Input: part model. Units: mm. Frame: model coordinates. Face numbers are marked on the shaded views. Give positions to 0.01 mm unless a question says otherwise; leave off trailing zeros. Loops run counter-clockwise (first coordinate to the right, second up) from the corner with the lowest first, then second, coordinate; pieces in that order, holes last. Notation, with made-up numbers: (32.5, 57.25) -> (71.5, 57.25) arc R29 cw to (71.5, 90.25) -> close; hole circle Ø5 at (-16, -27.75). An arc over 180 degrees is marked (long way). Answer in a Markdown table with one row per item. Add a question column.
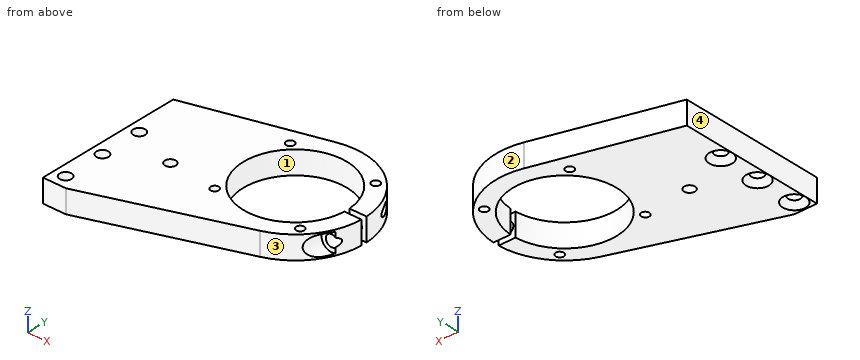
```python
from build123d import *

# Parameters (mm, degrees)
BOSS_EXTRUDE1_DEPTH         = 12.7
CUT_EXTRUDE1_DEPTH          = 13.7
SKETCH3_W                   = 28.575
SKETCH3_H                   = 12.7
F_8_CLEARANCE_HOLE1_D       = 4.5
F_8_CLEARANCE_HOLE1_DEPTH   = 12.7
F_1_4_CLEARANCE_HOLE1_D     = 6.6
F_1_4_CLEARANCE_HOLE1_DEPTH = 12.7
F_12_CLEARANCE_HOLE1_D      = 6
F_12_CLEARANCE_HOLE1_DEPTH  = 12.7
HOLE1_D                     = 6.4
HOLE1_DEPTH                 = 24.77643101
HOLE1_CBORE_D               = 11.2
HOLE1_CBORE_DEPTH           = 11.77643101
F_10_CLEARANCE_HOLE1_D      = 5
F_10_CLEARANCE_HOLE1_DEPTH  = 36.4125
CHAMFER1_SIZE               = 3
SKETCH14_R                  = 4
SKETCH14_R_2                = 3
BOSS_EXTRUDE2_DEPTH         = 12.7


with BuildPart() as part:
    # Sketch1 → Boss-Extrude1 (new body)
    with BuildSketch(Plane(origin=(0, 0, 0), x_dir=(-1, 0, 0), z_dir=(0, 0, -1))):
        with BuildLine():
            Line((224.169455465, 127.72254562), (151.435240745, 147.211619716))
            ThreePointArc((151.435240745, 147.211619716), (105.257753851, 121.607458019), (129.246532787, 74.570537656))
            Line((129.246532787, 74.570537656), (211.469455465, 46.304993078))
            Line((211.469455465, 46.304993078), (224.169455465, 46.304993078))
            Line((224.169455465, 46.304993078), (224.169455465, 127.72254562))
        make_face()
    extrude(amount=-BOSS_EXTRUDE1_DEPTH)

    # Sketch2 → Cut-Extrude1 (cut, through all)
    with BuildSketch(Plane.XY.offset(12.7)):
        with BuildLine():
            Line((-103.633291463, 112.093938317), (-113.179018515, 112.093938317))
            ThreePointArc((-113.179018515, 112.093938317), (-113.134717032, 110.506438317), (-113.179018515, 108.918938317))
            Line((-113.179018515, 108.918938317), (-103.633291463, 108.918938317))
            ThreePointArc((-103.633291463, 108.918938317), (-103.600117032, 110.506438317), (-103.633291463, 112.093938317))
        make_face()
    extrude(amount=-CUT_EXTRUDE1_DEPTH, mode=Mode.SUBTRACT)

    # Sketch3 → Cut-Revolve1 (revolve, cut)
    with BuildSketch(Plane(origin=(0, 110.506438317, 0), x_dir=(1, 0, 0), z_dir=(0, 1, 0))):
        with Locations((-127.312617032, -6.35)):
            Rectangle(SKETCH3_W, SKETCH3_H)
    revolve(axis=Axis((-141.600117032, 110.506438317, 0), (0, 0, 1)), mode=Mode.SUBTRACT)

    # #8 Clearance Hole1
    with Locations(Plane.XY.offset(12.7)):
        with Locations((-117.978117032, 86.884438317), (-165.222117032, 86.884438317), (-165.222117032, 134.128438317), (-117.978117032, 134.128438317)):
            Hole(F_8_CLEARANCE_HOLE1_D / 2, depth=F_8_CLEARANCE_HOLE1_DEPTH)

    # 1/4 Clearance Hole1
    with Locations(Plane(origin=(0, 0, 0), x_dir=(-1, 0, 0), z_dir=(0, 0, -1))):
        with Locations((217.819455465, 53.304993078), (217.819455465, 76.304993078), (217.819455465, 99.304993078)):
            Hole(F_1_4_CLEARANCE_HOLE1_D / 2, depth=F_1_4_CLEARANCE_HOLE1_DEPTH)

    # #12 Clearance Hole1
    with Locations(Plane.XY.offset(12.7)):
        with Locations((-192.169455465, 89.72254562)):
            Hole(F_12_CLEARANCE_HOLE1_D / 2, depth=F_12_CLEARANCE_HOLE1_DEPTH)

    # Hole1
    with Locations(Plane(origin=(0, 84.142507307, 0), x_dir=(-1, 0, 0), z_dir=(0, -1, 0))):
        with Locations((108.633291463, -6.35)):
            CounterBoreHole(HOLE1_D / 2, HOLE1_CBORE_D / 2, HOLE1_CBORE_DEPTH, depth=HOLE1_DEPTH)

    # #10 Clearance Hole1
    with Locations(Plane(origin=(0, 112.093938317, 0), x_dir=(-1, 0, 0), z_dir=(0, -1, 0))):
        with Locations((108.633291463, -6.35)):
            Hole(F_10_CLEARANCE_HOLE1_D / 2, depth=F_10_CLEARANCE_HOLE1_DEPTH)

    # Chamfer1
    chamfer1_edges = [part.edges().sort_by_distance(p)[0] for p in [
        (-221.119455465, 99.304993078, 0),
        (-221.119455465, 76.304993078, 0),
        (-221.119455465, 53.304993078, 0),
    ]]
    chamfer(chamfer1_edges, length=CHAMFER1_SIZE)

    # Sketch14 → Boss-Extrude2 (add)
    with BuildSketch(Plane(origin=(0, 0, 0), x_dir=(-1, 0, 0), z_dir=(0, 0, -1))):
        with Locations((192.169455465, 89.72254562)):
            Circle(SKETCH14_R)
        with Locations((192.169455465, 89.72254562)):
            Circle(SKETCH14_R_2, mode=Mode.SUBTRACT)
    extrude(amount=-BOSS_EXTRUDE2_DEPTH)


solid = part.part
```
1) Pull-direction query (X, two-part tool) for the marked faces 1, 2, 3 and 4; classes: +X half, -X half, draft (parallel to the pull), parting line (faces both ways), or undercut.
2) Section B-B on z = 6.35. State how many separate pieces and enclosed holes the cut face has, and give its area (3 significant figures).
3) Pin query (flat end, axial travel): pin 1 (2 mm diameter, centred on y = 117.5, z = 8, fed in from +X); pin 2 (8.5 mm diameter, centred on x = -217.82, y = 99.3, fed in from -Z) (3 decimals); pin 3 (10.5 mm diameter, centred on x = -217.82, y = 76.3, fed in from -Z) (3 decimals); pin 4 (6 mm diameter, centred on x = -165.22, y = 86.88, fed in from +Z). Return the tip coordinate at first contact, or that it passes through.
4) Section C-C on x = -192. Output: boundary loops of the cut face in (y, z), and give its area (3 significant figures).
5) Section D-D on y = 63. Output: boundary loops of the cut face in (x, z), and give its area (3 significant figures).
6) Material intervals for line 1 along Y through (x, z) = (-116, 1.25); line 2 along X through (y, z) = (115.5, 4.5); line 3 along X through (y, z) = (87.5, 4.25), sorted ascending.
7) Section A-A on y = 114. Output: boundary loops of the cut face in (x, z), and give its area (3 significant figures).
Working result:
| question | item | result |
|---|---|---|
| 1 | face 1 | undercut |
| 1 | face 2 | parting line |
| 1 | face 3 | +X half |
| 1 | face 4 | -X half |
| 2 | separate pieces | 3 |
| 2 | enclosed holes | 8 |
| 2 | area | 6,060 mm2 |
| 3 | pin 1 | stops at x = -104.08 |
| 3 | pin 2 | stops at z = 2.045 |
| 3 | pin 3 | stops at z = 1.045 |
| 3 | pin 4 | stops at z = 12.7 |
| 4 | outline | (53, 0) -> (86.73, 0) -> (86.73, 12.7) -> (53, 12.7) -> close; (92.72, 0) -> (136.34, 0) -> (136.34, 12.7) -> (92.72, 12.7) -> close |
| 4 | area | 982 mm2 |
| 5 | outline | (-224.17, 0) -> (-162.9, 0) -> (-162.9, 12.7) -> (-224.17, 12.7) -> close |
| 5 | area | 778 mm2 |
| 6 | line 1 | y = 82.42 to 85.81, 87.96 to 97.81, 123.2 to 133.06, 135.2 to 138.59 |
| 6 | line 2 | x = -224.17 to -169.74, -113.46 to -110.31, -106.95 to -103.93 |
| 6 | line 3 | x = -224.17 to -194.18, -190.15 to -167.39, -163.06 to -158.55, -124.65 to -120.14, -115.81 to -113.82 |
| 7 | outline | (-224.17, 0) -> (-169.96, 0) -> (-169.96, 12.7) -> (-224.17, 12.7) -> close; (-113.24, 0) -> (-103.76, 0) -> (-103.76, 12.7) -> (-113.24, 12.7) -> close; hole circle Ø5 at (-108.63, 6.35) |
| 7 | area | 789 mm2 |
